Design review of the part built by this model. Coordinates are the model's own, in mm. Face numbers are marked on the shaded views. A direction names the side the tool comes from. Round coordinates to 2 decimals unless told otherwise and drop trailing zeros. Loops run counter-clockwise (first coordinate to the right, second up) from the corner with the lowest first, then second, coordinate; pieces in that order, holes last. Notation, with made-up numbers: (64.5, 78) - (71.5, 78) arc R21 ccw to (71.5, 113) - close; hole circle Ø11 at (-30, 55). An arc over 180 degrees is marked (long way). Use one line per item in the form item = value. Start each with the question number.
(1) Machinability: for the marked faces 4 and 5, which of the approach directions +Z, -Z, +X, -X, +Y, -Y give a long, thin tool a straight path to every point of the face, cutting with its end or side? Answer none if there is none.
(2) For pin 1 (8 mm diameter, centred on x = -53, z = -9.5, fed in from +Y); pin 2 (7.5 mm diameter, centred on x = 83.15, z = 0, fed in from -Y); pin 3 (2 mm diameter, centred on y = 98.5, z = 56, fed in from -X); pin 4 (3.5 mm diameter, centred on x = -83.15, z = 0, fed in from -Y), all flat-tipped, find the tip position at first contact; note any pin that passes through.
(3) Wall thickness on probe 1 along Y at (x, z) = (71.5, 46); probe 2 along Y at (x, z) = (13, -5.5); probe 3 along Z at (x, y) = (-45, 42): over which ranges is each line inside the solid? List them lowest first. Write a range as [from, to].
(4) We need section A-A, the plane z = 0. Write out the cut boundary in (x, y).
(5) The part is to be moulded in two halves that separate along Z. For the marked faces 1, 2 and 3, say which applies: released by +Z, released by -Z, zero draft, split by the parting line, or undercut.
(6) We need section B-B, the plane x = 0. Write out the cut boundary in (y, z), then the cut area to 3 significant figures.
(7) We need section D-D, the plane z = 83.15. Write out the cut boundary in (x, y), then the cut area to 3 significant figures.
(8) We need section C-C, the plane x = -83.15. Write out the cut boundary in (y, z).
from build123d import *

# Parameters (mm, degrees)
F_4_6_4_6_DIAMETER_HOLE1_D = 4.6


with BuildPart() as part:
    # Sketch1 → Revolve1 (revolve)
    with BuildSketch(Plane.XY, mode=Mode.PRIVATE) as revolve1_sk:
        with BuildLine():
            Line((0, 99.4), (56.3, 99.4))
            ThreePointArc((56.3, 99.4), (66.9, 110), (77.5, 99.4))
            Line((77.5, 99.4), (88.25, 99.4))
            Line((88.25, 99.4), (88.25, 95.4))
            Line((88.25, 95.4), (70.75, 95.4))
            Line((70.75, 95.4), (58.585106664, 50))
            Line((58.585106664, 50), (60, 50))
            Line((60, 50), (60, 0))
            Line((60, 0), (0, 0))
            Line((0, 0), (0, 99.4))
        make_face()
    revolve(revolve1_sk.sketch.rotate(Axis((0, -46.308457921, 0), (0, 1, 0)), 90), axis=Axis((0, -46.308457921, 0), (0, 1, 0)))

    # Ø4.6 (4.6) Diameter Hole1 (through all)
    with Locations(Plane(origin=(0, 99.4, 0), x_dir=(1, 0, 0), z_dir=(0, 1, 0))):
        with Locations((0, -83.15), (-83.15, 0), (0, 83.15), (83.15, 0)):
            Hole(F_4_6_4_6_DIAMETER_HOLE1_D / 2)


solid = part.part
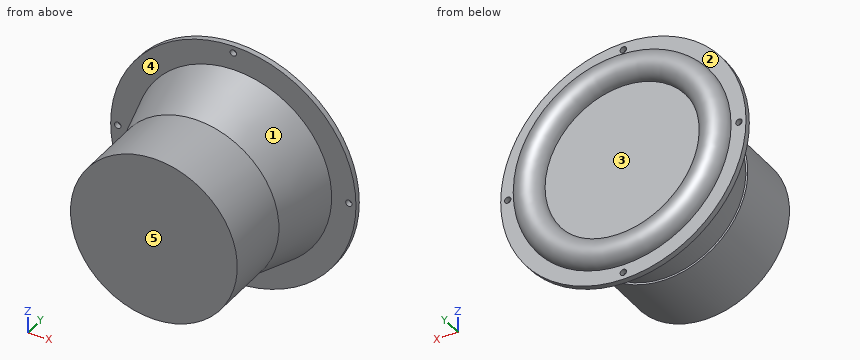
Data:
q1.face_4 = -Y
q1.face_5 = +Z, -Z, +X, -X, -Y
q2.pin_1 = 104.91
q2.pin_2 = 95.4
q2.pin_3 = -69.01
q2.pin_4 = through
q3.probe_1 = [95.4, 99.4]
q3.probe_2 = [0, 99.4]
q3.probe_3 = [-39.69, 39.69]
q4.outline = (-88.25, 95.4) - (-85.45, 95.4) - (-85.45, 99.4) - (-88.25, 99.4) - close; (-80.85, 95.4) - (-70.75, 95.4) - (-58.59, 50) - (-60, 50) - (-60, 0) - (60, 0) - (60, 50) - (58.59, 50) - (70.75, 95.4) - (80.85, 95.4) - (80.85, 99.4) - (77.5, 99.4) arc R10.6 ccw to (56.3, 99.4) - (-56.3, 99.4) arc R10.6 ccw to (-77.5, 99.4) - (-80.85, 99.4) - close; (85.45, 95.4) - (88.25, 95.4) - (88.25, 99.4) - (85.45, 99.4) - close
q5.face_1 = split by the parting line
q5.face_2 = zero draft
q5.face_3 = undercut
q6.outline = (0, -60) - (50, -60) - (50, -58.59) - (95.4, -70.75) - (95.4, -80.85) - (99.4, -80.85) - (99.4, -77.5) arc R10.6 ccw to (99.4, -56.3) - (99.4, 56.3) arc R10.6 ccw to (99.4, 77.5) - (99.4, 80.85) - (95.4, 80.85) - (95.4, 70.75) - (50, 58.59) - (50, 60) - (0, 60) - close; (95.4, -88.25) - (99.4, -88.25) - (99.4, -85.45) - (95.4, -85.45) - close; (95.4, 85.45) - (99.4, 85.45) - (99.4, 88.25) - (95.4, 88.25) - close
q6.area = 12,900 mm^2
q7.outline = (-29.57, 95.4) - (-2.3, 95.4) - (-2.3, 99.4) - (-29.57, 99.4) - close; (2.3, 95.4) - (29.57, 95.4) - (29.57, 99.4) - (2.3, 99.4) - close
q7.area = 218 mm^2
q8.outline = (95.4, -29.57) - (99.4, -29.57) - (99.4, -2.3) - (95.4, -2.3) - close; (95.4, 2.3) - (99.4, 2.3) - (99.4, 29.57) - (95.4, 29.57) - close
